Here's how the part is built. I have some questions about the finished solid (model axes, mm). Face numbers are marked on the shaded views. Coordinates: 2 decimals unless noted, no trailing zeros. Write each loop counter-clockwise with the first axis right and the second up, starting at its lowest first coordinate (ties: lowest second). Pieces come first, ordered by that corner, then holes. Notation, with made-up numbers: (-29.75, -26.75) -> (-6.75, -26.75) arc R10 cw to (-6.75, -21.75) -> close; hole circle Ø9 at (11, 29). An arc over 180 degrees is marked (long way). Use a Markdown table: item, result. Add a question column.
Item 1: Imagine slicing it at D-D, the plane x = 17.5. Write out the boundary of the cut face in (y, z).
Item 2: If we mould it in two halves opening along X, with no side actions, what happens to the marked faces 1, 2 and 3? For each: pulls with the +X half, pulls with the -X half, needs draft (parallel to the pull), parting line crosses it, or undercut.
Item 3: Imagine slicing it at A-A, the plane z = 22. Write out the boundary of the cut face in (x, y).
Item 4: If I drill on line 1 along Z through (x, y) = (75.5, 1.2); line 2 along X through (y, z) = (3.85, 52.5); line 3 along X through (y, z) = (0.55, 42.5), over which ranges is the centre line in solid material (lowest first)? Write a range as from..to.
Item 5: Will this pin go through, and if not, where does the flat tip stop? pin 1 Ø2.5 at (x, z) = (40.75, 42.42) entering from +Y.
Item 6: Imagine slicing it at C-C, the plane y = 1.75. Count the separate pieces of the cut face and the enclosed holes in it, and give its area (3 significant figures).
Item 7: Imagine slicing it at B-B, the plane x = 60. Write out the boundary of the cut face in (y, z).
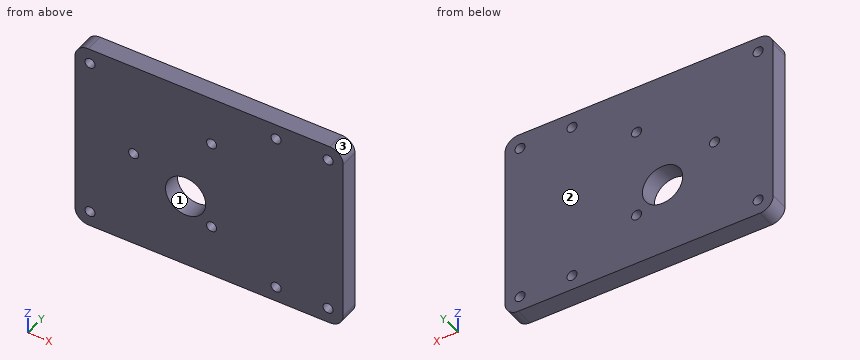
Autodesk Inventor part; units mm, degrees
ref_plane "YZ Plane" through (0, 0, 0) normal (1, 0, 0) x (0, 1, 0)
ref_plane "XZ Plane" through (0, 0, 0) normal (0, 1, 0) x (-1, 0, 0)
ref_plane "XY Plane" through (0, 0, 0) normal (0, 0, 1) x (1, 0, 0)
sketch "スケッチ1" plane through (0, 0, 0) normal (0, 1, 0) x (-1, 0, 0)
  line L0 (0, 0) -> (-80, 0)
  line L1 (-80, 0) -> (-80, 57)
  line L2 (-80, 57) -> (0, 57)
  line L3 (0, 57) -> (0, 0)
  dimension "d2" = 80
  dimension "d3" = 57
extrude "押し出し1" add sketch "スケッチ1" along normal blind 5.5
sketch "スケッチ2" plane through (0, 0, 0) normal (0, -1, 0) x (1, 0, 0)
  line L0 (80, 0) -> (0, 0)
  line L1 (80, 57) -> (80, 0)
  line L2 (0, 0) -> (0, 57)
  line L3 (0, 57) -> (80, 57)
  point P0 (75.5, 4.5)
  point P1 (4.5, 4.5)
  point P2 (4.5, 52.5)
  point P3 (75.5, 52.5)
  dimension "d4" = 4.5
  dimension "d5" = 4.5
  dimension "d6" = 4.5
  dimension "d7" = 4.5
  dimension "d8" = 4.5
  dimension "d9" = 4.5
  dimension "d10" = 4.5
  dimension "d11" = 4.5
hole "穴1" at (75.5, 0, 4.5) at (4.5, 0, 4.5) at (4.5, 0, 52.5) at (75.5, 0, 52.5) direction (0, 1, 0) diameter 3 end through all
fillet "フィレット1" radius 4 4 edges at (80, 2.75, 0) (0, 2.75, 0) (80, 2.75, 57) (0, 2.75, 57)
sketch "スケッチ3" plane through (0, 0, 0) normal (0, -1, 0) x (1, 0, 0)
  circle A0 centre (33, 29) radius 15.5
  line L0 (0, 4) -> (0, 53)
  line L1 (80, 53) -> (80, 4)
  line L2 (4, 57) -> (76, 57)
  line L3 (33, 29) -> (17.5, 29)
  line L4 (33, 29) -> (40.75, 15.5766)
  line L5 (33, 29) -> (40.75, 42.4234)
  point P0 (0, 0)
  dimension "d20" = 31
  dimension "d21" = 80
  dimension "d22" = 47
  dimension "d23" = 28
  dimension "d24" = 120
  dimension "d25" = 120
hole "穴2" at (40.75, 0, 15.5766) at (40.75, 0, 42.4234) at (17.5, 0, 29) direction (0, 1, 0) diameter 3 end through all
sketch "スケッチ4" plane through (0, 0, 0) normal (0, -1, 0) x (1, 0, 0)
  circle A0 centre (33, 22) radius 6
  line L0 (80, 53) -> (80, 4)
  line L1 (4, 57) -> (76, 57)
  point P0 (0, 0)
  dimension "d33" = 12
  dimension "d34" = 47
  dimension "d35" = 35
extrude "押し出し2" cut sketch "スケッチ4" against normal through all
sketch "スケッチ5" plane through (0, 5.5, 0) normal (0, 1, 0) x (1, 0, 0)
  line L0 (4, -57) -> (76, -57)
  line L1 (80, -53) -> (80, -4)
  line L2 (76, 0) -> (4, 0)
  point P0 (0, 0)
  point P1 (60, -52.5)
  point P2 (60, -4.5)
  dimension "d38" = 4.5
  dimension "d39" = 20
  dimension "d40" = 20
  dimension "d41" = 4.5
hole "穴3" at (60, 5.5, 52.5) at (60, 5.5, 4.5) direction (0, -1, 0) diameter 3 end through all
properties part number "上下直動t5.5" material "木材 (カエデ材)"
Ans:
| question | item | result |
|---|---|---|
| 1 | outline | (0, 0) -> (5.5, 0) -> (5.5, 27.5) -> (0, 27.5) -> close; (0, 30.5) -> (5.5, 30.5) -> (5.5, 57) -> (0, 57) -> close |
| 2 | face 1 | undercut |
| 2 | face 2 | needs draft |
| 2 | face 3 | pulls with the +X half |
| 3 | outline | (0, 0) -> (27, 0) -> (27, 5.5) -> (0, 5.5) -> close; (39, 0) -> (80, 0) -> (80, 5.5) -> (39, 5.5) -> close |
| 4 | line 1 | z = 0..3, 6..51, 54..57 |
| 4 | line 2 | x = 0..3, 6..58.5, 61.5..74, 77..80 |
| 4 | line 3 | x = 0..39.25, 42.25..80 |
| 5 | pin 1 | passes through |
| 6 | separate pieces | 1 |
| 6 | enclosed holes | 10 |
| 6 | area | 4,370 mm^2 |
| 7 | outline | (0, 0) -> (5.5, 0) -> (5.5, 3) -> (0, 3) -> close; (0, 6) -> (5.5, 6) -> (5.5, 51) -> (0, 51) -> close; (0, 54) -> (5.5, 54) -> (5.5, 57) -> (0, 57) -> close |
